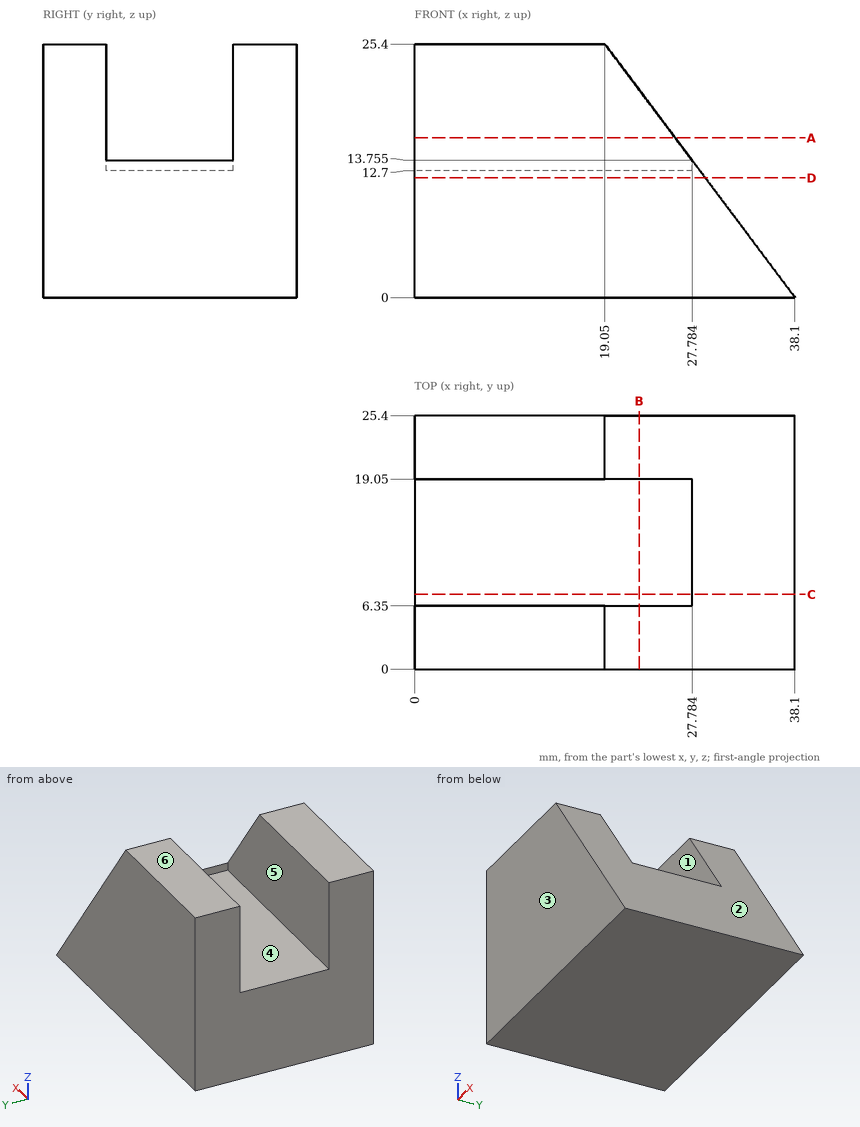
The figure shows three views and two pictorial views of one solid part (mm, origin at its lowest corner). Answer the questions. A direction names the side the tool comes from. Coordinates: 2 decimals unless noted, no trailing zeros. Loops run counter-clockwise (first coordinate to the right, second up) from the corner with the lowest first, then second, coordinate; pieces in that order, holes last. Notation, with made-up numbers: (7, 34.25) - (27, 34.25) arc R8 cw to (27, 40.25) - close; hole circle Ø8 at (7.5, 84). An arc over 180 degrees is marked (long way). Use a Markdown table: item, result. Add a question column.
1) For the marked faces 1 and 2, determine the directions among +Z, -Z, +X, -X, +Y, -Y from which every point of the face is accessible in a straight line to the end or side of a thin tool.
2) The mould has two halves that part along Y. Classify the marked faces 3, 4, 5 and 6: released by +Y, released by -Y, zero draft, split by the parting line, or undercut.
3) Given pin 1 (1 mm diameter, centred on x = 32, y = 2.5, fed in from +Z); pin 2 (1 mm diameter, centred on x = 32.5, y = 4.5, fed in from +Z); pin 3 (1.5 mm diameter, centred on x = 28.5, y = 10, fed in from +Z) (3 decimals), each flat-ended and moving along its own axis, determine where each tip first touches the part or whether it passes through.
4) The part is cut by section C-C, the plane y = 7.5. Give the vertices of the cut face in (x, z) (3 decimals), and give its area (3 significant figures).
5) The part is cut by section B-B, the plane x = 22.5. Give the vertices of the cut face in (y, z).
6) The part is cut by section A-A, the plane z = 16. Give the vertices of the cut face in (x, y).
7) Find the intervals of material crossed by line 1 (Y direction, x = 6.5, z = 17); line 2 (Z direction, x = 5, y = 7.5); line 3 (Z direction, x = 35, y = 9), in increasing order.
8) The part is cut by section D-D, the plane z = 12. Give the vertices of the cut face in (x, y).
Here are the results:
| question | item | result |
|---|---|---|
| 1 | face 1 | +Z, -X |
| 1 | face 2 | +Z, +X, +Y, -Y |
| 2 | face 3 | released by -Y |
| 2 | face 4 | undercut |
| 2 | face 5 | undercut |
| 2 | face 6 | zero draft |
| 3 | pin 1 | stops at z = 8.8 |
| 3 | pin 2 | stops at z = 8.13 |
| 3 | pin 3 | stops at z = 13.755 |
| 4 | outline | (0, 0) - (38.1, 0) - (27.784, 13.755) - (27.784, 12.7) - (0, 12.7) - close |
| 4 | area | 424 mm^2 |
| 5 | outline | (0, 0) - (25.4, 0) - (25.4, 20.8) - (19.05, 20.8) - (19.05, 12.7) - (6.35, 12.7) - (6.35, 20.8) - (0, 20.8) - close |
| 6 | outline | (0, 0) - (26.1, 0) - (26.1, 6.35) - (0, 6.35) - close; (0, 19.05) - (26.1, 19.05) - (26.1, 25.4) - (0, 25.4) - close |
| 7 | line 1 | y = 0 to 6.35, 19.05 to 25.4 |
| 7 | line 2 | z = 0 to 12.7 |
| 7 | line 3 | z = 0 to 4.13 |
| 8 | outline | (0, 0) - (29.1, 0) - (29.1, 25.4) - (0, 25.4) - close |
